Source: CAD feature listing. Evaluate the final solid. Frame: model axes, mm. Face numbers are marked on the shaded views. A direction names the side the tool comes from. Round coordinates to 2 decimals unless told otherwise and drop trailing zeros. Loops run counter-clockwise (first coordinate to the right, second up) from the corner with the lowest first, then second, coordinate; pieces in that order, holes last. Notation, with made-up numbers: M 69,-24.5 L 95,-24.5 A17 ccw 95,-8.5 Z; hole C 65.5,-12.5 d4. An arc over 180 degrees is marked long. Answer as a JSON object with one key per item and string values.
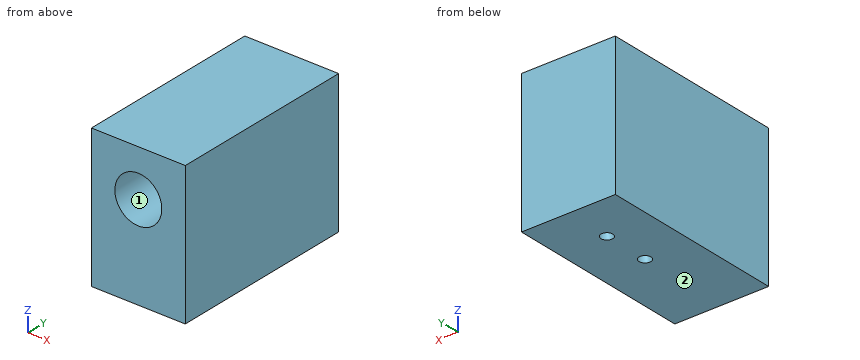
Autodesk Inventor part; units mm, degrees
ref_plane "YZ Plane" through (0, 0, 0) normal (1, 0, 0) x (0, 1, 0)
ref_plane "XZ Plane" through (0, 0, 0) normal (0, 1, 0) x (-1, 0, 0)
ref_plane "XY Plane" through (0, 0, 0) normal (0, 0, 1) x (1, 0, 0)
sketch "Sketch1" plane through (0, 0, 0) normal (0, 1, 0) x (-1, 0, 0)
  circle A0 centre (3.4811, 6.9947) radius 6.35
  line L0 (-9.2189, 19.6947) -> (16.1811, 19.6947)
  line L1 (16.1811, 19.6947) -> (16.1811, -18.4053)
  line L2 (16.1811, -18.4053) -> (-9.2189, -18.4053)
  line L3 (-9.2189, -18.4053) -> (-9.2189, 19.6947)
  point P0 (0, 0)
  dimension "d0" = 12.7
  dimension "d1" = 25.4
  dimension "d2" = 38.1
  dimension "d3" = 12.7
  dimension "d4" = 12.7
extrude "Extrusion1" add sketch "Sketch1" along normal blind 50.8 contours A0 | L0 L1 L2 L3
extrude "Extrusion4" cut sketch "Sketch1" along normal blind 44.45 contours A0
sketch "Sketch3" plane through (9.2189, 0, -18.4053) normal (0, 0, -1) x (-1, 0, 0)
  line L0 (25.4, 0) -> (0, 0)
  line L1 (12.7, 0) -> (12.7, 50.8)
  line L2 (0, 50.8) -> (25.4, 50.8)
  circle A0 centre (12.7, 25.4) radius 1.5875
  circle A1 centre (12.7, 38.1) radius 1.5875
  point P0 (9.2189, 0)
  dimension "d23" = 3.175
  dimension "d24" = 3.175
  dimension "d25" = 25.4
  dimension "d26" = 12.7
extrude "Extrusion5" cut sketch "Sketch3" against normal blind 12.7 contours A0 L1 | L1 A0
sketch "Sketch4" plane through (9.2189, -0.0789, -18.4053) normal (0, 0, -1) x (-1, 0, 0)
  line L0 (25.4, 0) -> (0, 0)
  line L1 (12.7, 0) -> (12.7, 50.8)
  line L2 (0, 50.8) -> (25.4, 50.8)
  circle A0 centre (12.7, 25.4) radius 1.5875
  circle A1 centre (12.7, 38.1) radius 1.5875
  point P0 (9.2189, 0)
  point P1 (12.7, 39.6875)
  point P2 (12.7, 36.5125)
  dimension "d30" = 3.175
  dimension "d31" = 3.175
  dimension "d32" = 25.4
  dimension "d29" = 12.7
extrude "Extrusion6" cut sketch "Sketch4" against normal blind 25.4 contours A1 L1 | L1 A1
properties part number "Cylinder"
Item 1: Access query for the marked faces 1 and 2. Directions: +Z, -Z, +X, -X, +Y, -Y. A direction counts if a zero-diameter tool reaches every point of the face in a straight line with its end or side. Return the directions, or none.
Answer sheet:
{"face 1": "-Y", "face 2": "-Z, +X, -X, +Y, -Y"}
Item 2: Section A-A on x = -4. Return the cut outline in (y, z).
Answer sheet:
{"outline": "M 0,-18.41 L 23.9,-18.41 L 23.9,-5.71 L 26.9,-5.71 L 26.9,-18.41 L 36.52,-18.41 L 36.52,0.67 L 0,0.67 Z; M 0,13.32 L 44.45,13.32 L 44.45,0.67 L 39.52,0.67 L 39.52,-18.41 L 50.8,-18.41 L 50.8,19.69 L 0,19.69 Z"}
Item 3: Section C-C on x = 1.25. Return the cut outline in (y, z).
Answer sheet:
{"outline": "M 0,-18.41 L 50.8,-18.41 L 50.8,19.69 L 0,19.69 L 0,11.23 L 44.45,11.23 L 44.45,2.76 L 0,2.76 Z"}
Item 4: Section D-D on y = 25.4. Return the cut outline in (x, z), then the cut area to 3 significant figures.
Answer sheet:
{"outline": "M -16.18,-18.41 L -5.07,-18.41 L -5.07,-5.71 L -1.89,-5.71 L -1.89,-18.41 L 9.22,-18.41 L 9.22,19.69 L -16.18,19.69 Z; hole C -3.48,6.99 d12.7", "area": "801 mm²"}
Item 5: Line query: probe 1 along X at (y, z) = (25.4, -14.25); probe 2 along Y at (x, z) = (-7.75, 3.5); probe 3 along X at (y, z) = (25, -9). Output: solid intervals per line, ascending. Write a range as from..to.
Answer sheet:
{"probe 1": "x = -16.18..-5.07, -1.89..9.22", "probe 2": "y = 44.45..50.8", "probe 3": "x = -16.18..-5.02, -1.94..9.22"}
Item 6: Section B-B on y = 20. Return the cut outline in (x, z), then the cut area to 3 significant figures.
Answer sheet:
{"outline": "M -16.18,-18.41 L 9.22,-18.41 L 9.22,19.69 L -16.18,19.69 Z; hole C -3.48,6.99 d12.7", "area": "841 mm²"}
Item 7: Contact query for flat-ended pins moving along their axis: pin 1 Ø4 at (x, y) = (-3.48, 38.02) entering from -Z; pin 2 Ø4 at (x, z) = (-4.5, 6) entering from -Y. Output: stop coordinate, or through.
Answer sheet:
{"pin 1": "stops at z = -18.41", "pin 2": "stops at y = 44.45"}
